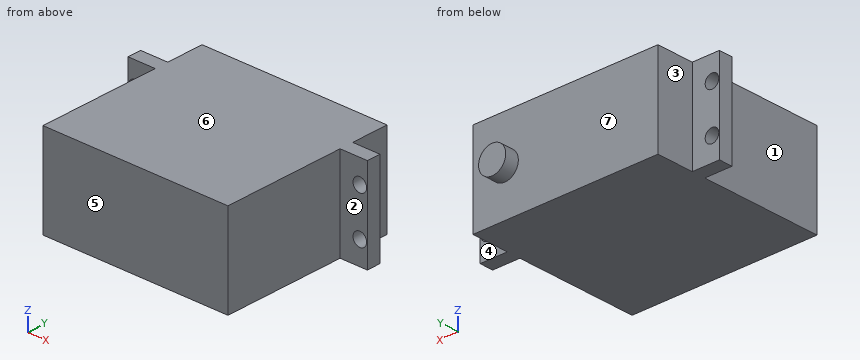
from build123d import *

# Parameters (mm, degrees)
BOSS_EXTRUDE1_DEPTH = 20.1
SKETCH2_R           = 3
BOSS_EXTRUDE2_DEPTH = 3
CUT_EXTRUDE1_REACH  = 61.011
SKETCH3_R           = 1.5


with BuildPart() as part:
    # Sketch1 → Boss-Extrude1 (new body)
    with BuildSketch(Plane.XY):
        Polygon((0, 0), (40.8, 0), (40.8, 26.8), (46.8, 26.8), (46.8, 29.8), (40.8, 29.8), (40.8, 38), (0, 38), (0, 29.8), (-6, 29.8), (-6, 26.8), (0, 26.8), align=None)
    extrude(amount=BOSS_EXTRUDE1_DEPTH)

    # Sketch2 → Boss-Extrude2 (add)
    with BuildSketch(Plane(origin=(0, 38, 0), x_dir=(1, 0, 0), z_dir=(0, 1, 0))):
        with Locations((33.8, -10.05)):
            Circle(SKETCH2_R)
    extrude(amount=BOSS_EXTRUDE2_DEPTH)

    # Sketch3 → Cut-Extrude1 (cut, up to next)
    with BuildSketch(Plane(origin=(0, 29.8, 0), x_dir=(1, 0, 0), z_dir=(0, 1, 0)), mode=Mode.PRIVATE) as cut_extrude1_sk1:
        with Locations(Location((45.15, -15.05, 0), (0, 0, 270))):
            Circle(SKETCH3_R)
    cut_extrude1_tool1 = extrude(cut_extrude1_sk1.sketch, amount=-CUT_EXTRUDE1_REACH, mode=Mode.PRIVATE) & part.part
    # Sketch3 → Cut-Extrude1 (cut, up to next)
    with BuildSketch(Plane(origin=(0, 29.8, 0), x_dir=(1, 0, 0), z_dir=(0, 1, 0)), mode=Mode.PRIVATE) as cut_extrude1_sk2:
        with Locations(Location((45.15, -5.05, 0), (0, 0, 270))):
            Circle(SKETCH3_R)
    cut_extrude1_tool2 = extrude(cut_extrude1_sk2.sketch, amount=-CUT_EXTRUDE1_REACH, mode=Mode.PRIVATE) & part.part
    # Sketch3 → Cut-Extrude1 (cut, up to next)
    with BuildSketch(Plane(origin=(0, 29.8, 0), x_dir=(1, 0, 0), z_dir=(0, 1, 0)), mode=Mode.PRIVATE) as cut_extrude1_sk3:
        with Locations(Location((-4.35, -5.05, 0), (0, 0, 270))):
            Circle(SKETCH3_R)
    cut_extrude1_tool3 = extrude(cut_extrude1_sk3.sketch, amount=-CUT_EXTRUDE1_REACH, mode=Mode.PRIVATE) & part.part
    # Sketch3 → Cut-Extrude1 (cut, up to next)
    with BuildSketch(Plane(origin=(0, 29.8, 0), x_dir=(1, 0, 0), z_dir=(0, 1, 0)), mode=Mode.PRIVATE) as cut_extrude1_sk4:
        with Locations(Location((-4.35, -15.05, 0), (0, 0, 270))):
            Circle(SKETCH3_R)
    cut_extrude1_tool4 = extrude(cut_extrude1_sk4.sketch, amount=-CUT_EXTRUDE1_REACH, mode=Mode.PRIVATE) & part.part
    add(cut_extrude1_tool1.solids().sort_by_distance((45.15, 29.8, 15.05))[0], mode=Mode.SUBTRACT)
    add(cut_extrude1_tool2.solids().sort_by_distance((45.15, 29.8, 5.05))[0], mode=Mode.SUBTRACT)
    add(cut_extrude1_tool3.solids().sort_by_distance((-4.35, 29.8, 5.05))[0], mode=Mode.SUBTRACT)
    add(cut_extrude1_tool4.solids().sort_by_distance((-4.35, 29.8, 15.05))[0], mode=Mode.SUBTRACT)


solid = part.part
Geometry: final body of the model. Coordinates: model frame, mm. Face numbers are marked on the shaded views. A direction names the side the tool comes from. Coordinates: 2 decimals unless noted, no trailing zeros. Loops run counter-clockwise (first coordinate to the right, second up) from the corner with the lowest first, then second, coordinate; pieces in that order, holes last. Notation, with made-up numbers: M 56,77 L 62,77 A19 ccw 62,83 Z; hole C 4.5,60.25 d2. An arc over 180 degrees is marked long. One line per item, written item: value. Start each with the question number.
1) Pin query (flat end, axial travel): P1, Ø1.8, axis at x = -4.35, z = 5.05, coming from the -Y side; P2, Ø8, axis at y = 5.5, z = 17.5, coming from the -X side; P3, Ø8, axis at x = 17.5, z = 10, coming from the +Y side; P4, Ø5, axis at x = -4.35, z = 15.05, coming from the -Y side. Return the tip coordinate at first contact, or that it passes through.
2) Reachability of the marked faces 1, 2, 3 and 4 from +Z, -Z, +X, -X, +Y, -Y: full face, straight path, thin tool, end or side. Return the list, or none.
3) Cut plane D-D (z = 10.05). Return loops of the section in (x, y), then the cut area to 3 significant figures.
4) Cut plane A-A (z = 15.05). Return loops of the section in (x, y).
5) Draft query along Y for the marked faces 5, 6 and 7. Return one class per face: released by +Y, released by -Y, zero draft, split by the parting line, or undercut.
6) Cut plane C-C (x = 33.8). Return loops of the section in (y, z), then the cut area to 3 significant figures.
7) Cut plane B-B (x = 45.15). Return loops of the section in (y, z).
8) Material intervals for L1, parallel to X at y = 28.15, z = 15.05; L2, parallel to Z at x = 45, y = 28; L3, parallel to Y at x = 22.5, z = 4, sorted ascending. Write a range as from..to.
Evaluation:
1. P1: through
1. P2: x = 0
1. P3: y = 38
1. P4: y = 26.8
2. face 1: +Z, -Z, -X, -Y
2. face 2: +Z, -Z, +X, -Y
2. face 3: +Z, -Z, -X, +Y
2. face 4: +Z, -Z, +X, +Y
3. outline: M -6,26.8 L 0,26.8 L 0,0 L 40.8,0 L 40.8,26.8 L 46.8,26.8 L 46.8,29.8 L 40.8,29.8 L 40.8,38 L 36.8,38 L 36.8,41 L 30.8,41 L 30.8,38 L 0,38 L 0,29.8 L -6,29.8 Z
3. area: 1,600 mm^2
4. outline: M -6,26.8 L -5.85,26.8 L -5.85,29.8 L -6,29.8 Z; M -2.85,26.8 L 0,26.8 L 0,0 L 40.8,0 L 40.8,26.8 L 43.65,26.8 L 43.65,29.8 L 40.8,29.8 L 40.8,38 L 0,38 L 0,29.8 L -2.85,29.8 Z; M 46.65,26.8 L 46.8,26.8 L 46.8,29.8 L 46.65,29.8 Z
5. face 5: released by -Y
5. face 6: zero draft
5. face 7: released by +Y
6. outline: M 0,0 L 38,0 L 38,7.05 L 41,7.05 L 41,13.05 L 38,13.05 L 38,20.1 L 0,20.1 Z
6. area: 782 mm^2
7. outline: M 26.8,0 L 29.8,0 L 29.8,3.55 L 26.8,3.55 Z; M 26.8,6.55 L 29.8,6.55 L 29.8,13.55 L 26.8,13.55 Z; M 26.8,16.55 L 29.8,16.55 L 29.8,20.1 L 26.8,20.1 Z
8. L1: -6..-5.85, -2.85..43.65, 46.65..46.8
8. L2: 0..3.56, 6.54..13.56, 16.54..20.1
8. L3: 0..38
